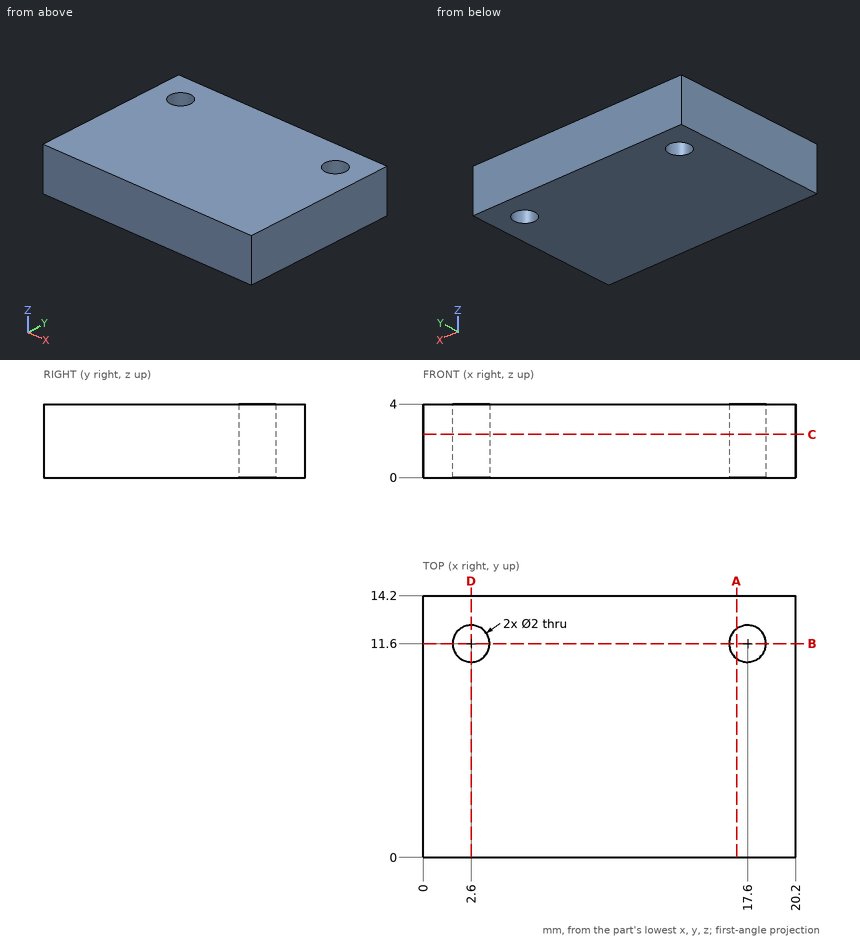
Input: dimensioned drawing with shaded views. Units: mm. Origin: part minimum x, y, z. Round coordinates to 2 decimals unless told otherwise and drop trailing zeros. Order: outer loops, then holes, each group sorted by start corner. A loop starts at its lowest first (then second) coordinate and runs counter-clockwise, first axis right, second up. Notation, with made-up numbers: (25, -32) -> (59, -32) arc R29 ccw to (59, -10) -> close; hole circle Ø1 at (23.5, 53.25). An arc over 180 degrees is marked (long way). Put each result on its own line as item: value. Start each with the question number.
Q1. First-contact query: pin 1 (1 mm diameter, centred on y = 10, z = 2.5, fed in from -X). Flat tip, straight axial feed; report the tip coordinate or a pass-through.
Q2. Section D-D on x = 2.6. Return the cut outline in (y, z), and give its area (3 significant figures).
Q3. Section A-A on x = 17. Return the cut outline in (y, z), and give its area (3 significant figures).
Q4. Section C-C on z = 2.35. Return the cut outline in (x, y).
Q5. Section B-B on y = 11.6. Return the cut outline in (x, z), and give its area (3 significant figures).
Q6. Line query: probe 1 along Y at (x, z) = (2.6, 1.95); probe 2 along Y at (x, z) = (3.5, 2.7); probe 3 along X at (y, z) = (10.75, 2). Output: solid intervals per line, ascending.
Ans:
1. pin 1: stops at x = 0
2. outline: (0, 0) -> (10.6, 0) -> (10.6, 4) -> (0, 4) -> close; (12.6, 0) -> (14.2, 0) -> (14.2, 4) -> (12.6, 4) -> close
2. area: 48.8 mm2
3. outline: (0, 0) -> (10.8, 0) -> (10.8, 4) -> (0, 4) -> close; (12.4, 0) -> (14.2, 0) -> (14.2, 4) -> (12.4, 4) -> close
3. area: 50.4 mm2
4. outline: (0, 0) -> (20.2, 0) -> (20.2, 14.2) -> (0, 14.2) -> close; hole circle Ø2 at (2.6, 11.6); hole circle Ø2 at (17.6, 11.6)
5. outline: (0, 0) -> (1.6, 0) -> (1.6, 4) -> (0, 4) -> close; (3.6, 0) -> (16.6, 0) -> (16.6, 4) -> (3.6, 4) -> close; (18.6, 0) -> (20.2, 0) -> (20.2, 4) -> (18.6, 4) -> close
5. area: 64.8 mm2
6. probe 1: y = 0 to 10.6, 12.6 to 14.2
6. probe 2: y = 0 to 11.16, 12.04 to 14.2
6. probe 3: x = 0 to 2.07, 3.13 to 17.07, 18.13 to 20.2
